```python
from build123d import *

# Parameters (mm, degrees)
SKETCH2_R           = 5.75
BOSS_EXTRUDE2_DEPTH = 10
SKETCH3_R           = 5
BOSS_EXTRUDE3_DEPTH = 17
SKETCH4_R           = 2.5
CUT_EXTRUDE1_DEPTH  = 10.7
SKETCH5_R           = 2.25
CUT_EXTRUDE2_DEPTH  = 17.7
CHAMFER4_SIZE       = 2
CHAMFER5_SIZE       = 0.5
CHAMFER6_SIZE       = 0.5


with BuildPart() as part:
    # Sketch2 → Boss-Extrude2 (new body)
    with BuildSketch(Plane.XY):
        with Locations((0, -0.068254458)):
            Circle(SKETCH2_R)
    extrude(amount=BOSS_EXTRUDE2_DEPTH)

    # Sketch3 → Boss-Extrude3 (add)
    with BuildSketch(Plane.XY.offset(10)):
        with Locations((0.02487522, 0)):
            Circle(SKETCH3_R)
    extrude(amount=BOSS_EXTRUDE3_DEPTH)

    # Sketch4 → Cut-Extrude1 (cut)
    with BuildSketch(Plane(origin=(0, 0, 0), x_dir=(-1, 0, 0), z_dir=(0, 0, -1))):
        Circle(SKETCH4_R)
    extrude(amount=-CUT_EXTRUDE1_DEPTH, mode=Mode.SUBTRACT)

    # Sketch5 → Cut-Extrude2 (cut)
    with BuildSketch(Plane.XY.offset(27)):
        with Locations((0, -0.093129678)):
            Circle(SKETCH5_R)
    extrude(amount=-CUT_EXTRUDE2_DEPTH, mode=Mode.SUBTRACT)

    # Chamfer4
    # the kernel refuses this chamfer: 2 mm, written as the material it takes off along each edge
    with BuildSketch(Plane(origin=(0, -0.068254458, 10), x_dir=(1, 0, 0), z_dir=(0, -1, 0))) as chamfer4_piece_1_section:
        Polygon((5.75, -CHAMFER4_SIZE), (5.75 - CHAMFER4_SIZE, 0), (5.75, 0), align=None)
    chamfer4_piece_1 = revolve(axis=Axis((0, -0.068254458, 10), (0, 0, 1)), mode=Mode.PRIVATE)
    chamfer4_piece_1 = chamfer4_piece_1 - Plane(origin=(0.02487522, 0, 8.408355985), x_dir=(1, 0, 0), z_dir=(0, 0, -1)) * Cylinder(5, 23, mode=Mode.PRIVATE)
    add(chamfer4_piece_1, mode=Mode.SUBTRACT)

    # Chamfer5
    chamfer5_edges = [part.edges().sort_by_distance(p)[0] for p in [
        (-4.97512478, 0, 27),
    ]]
    chamfer(chamfer5_edges, length=CHAMFER5_SIZE)

    # Chamfer6
    chamfer6_edges = [part.edges().sort_by_distance(p)[0] for p in [
        (-5.75, -0.068254458, 0),
    ]]
    chamfer(chamfer6_edges, length=CHAMFER6_SIZE)


solid = part.part
```
Model file for the job. Use its own axes, mm. A direction names the side the tool comes from. Give positions to 0.01 mm unless a question says otherwise; leave off trailing zeros. Write each loop counter-clockwise with the first axis right and the second up, starting at its lowest first coordinate (ties: lowest second). Pieces come first, ordered by that corner, then holes. Notation, with made-up numbers: M -7.5,34.25 L 50.5,34.25 A19 cw 50.5,69.25 Z; hole C 33,48 d9. An arc over 180 degrees is marked long. Use a Markdown table: item, result.
1) Pin check, flat tips, straight feed: pin 1 (2 mm diameter, centred on x = -4, y = 2.5, fed in from -Z); pin 2 (4 mm diameter, centred on y = 1, z = 13, fed in from -X); pin 3 (4 mm diameter, centred on y = -0.5, z = 17, fed in from +X); pin 4 (6 mm diameter, centred on x = -2, z = 11.5, fed in from +Y). Stop position of each tip, or through.
Responses:
| item | result |
|---|---|
| pin 1 | stops at z = 0 |
| pin 2 | stops at x = -4.98 |
| pin 3 | stops at x = 5.02 |
| pin 4 | stops at y = 5 |
2) Tool access for faces 1 (the cylindrical face through (0.54, -2.44, 5.28)), 2 (the flat face through (1, 2.1, 27)), 3 (the cylindrical face through (4.794, -1.502, 17.464)): list every direction of +Z, -Z, +X, -X, +Y, -Y with a clear straight run to the whole face (end or side of a thin tool).
Responses:
| item | result |
|---|---|
| face 1 | -Z |
| face 2 | +Z, +X, -X, +Y, -Y |
| face 3 | +Z |
3) Cut at A-A (z = 6.5). List the corners of the cut face in (x, y), and give its area (3 significant figures).
Responses:
| item | result |
|---|---|
| outline | C 0,-0.07 d11.5; hole C 0,0 d5 |
| area | 84.2 mm2 |
4) Drill centre lines: line 1 (Y direction, x = 0, z = 6); line 2 (Y direction, x = 0, z = 20); line 3 (X direction, y = -0.75, z = 14). Where is each one in solid material? Low to high. Write a range as from..to.
Responses:
| item | result |
|---|---|
| line 1 | y = -5.82..-2.5, 2.5..5.68 |
| line 2 | y = -5..-2.34, 2.16..5 |
| line 3 | x = -4.92..-2.15, 2.15..4.97 |
5) Pull direction X, two halves, no side cores. Call faces 4 (the cylindrical face through (-1.786, -1.462, 18.964)), 5 (the cylindrical face through (-1.25, -5.68, 4.2)), 6 (the flat face through (-2.4, -1.2, 0)): +X half, -X half, draft (parallel to the pull), parting line (faces both ways), or undercut.
Responses:
| item | result |
|---|---|
| face 4 | undercut |
| face 5 | parting line |
| face 6 | draft |
6) Cut at B-B (z = 18). List the corners of the cut face in (x, y), and give its area (3 significant figures).
Responses:
| item | result |
|---|---|
| outline | C 0.02,0 d10; hole C 0,-0.09 d4.5 |
| area | 62.6 mm2 |
